The model under review builds one solid part; all positions refer to its coordinate system, in mm. A direction names the side the tool comes from. Coordinates: 2 decimals unless noted, no trailing zeros. Order: outer loops, then holes, each group sorted by start corner. A loop starts at its lowest first (then second) coordinate and runs counter-clockwise, first axis right, second up. Notation, with made-up numbers: M -30.5,2 L -21.5,2 A6 ccw -21.5,9 Z; hole C 81.5,18 d5. An arc over 180 degrees is marked long. One line per item, written item: value.
```python
from build123d import *

# Parameters (mm, degrees)
SKETCH1_W           = 70
SKETCH1_H           = 40
BOSS_EXTRUDE1_DEPTH = 15
SKETCH2_R           = 7.5
CUT_EXTRUDE1_DEPTH  = 56.226805086
SKETCH3_R           = 11.5
CUT_EXTRUDE2_DEPTH  = 16.5
SKETCH4_R           = 2.6
CUT_EXTRUDE3_DEPTH  = 44.011626335
SKETCH5_W           = 10
SKETCH5_H           = 15
BOSS_EXTRUDE2_DEPTH = 3
SKETCH8_W           = 4.25
SKETCH8_H           = 15
BOSS_EXTRUDE5_DEPTH = 10
SKETCH9_W           = 0.6
SKETCH9_H           = 0.6
BOSS_EXTRUDE6_DEPTH = 10


with BuildPart() as part:
    # Sketch1 → Boss-Extrude1 (new body)
    with BuildSketch(Plane.XY):
        Rectangle(SKETCH1_W, SKETCH1_H)
    extrude(amount=BOSS_EXTRUDE1_DEPTH)

    # Sketch2 → Cut-Extrude1 (cut, through all)
    with BuildSketch(Plane.XZ.offset(20)):
        with Locations((-20, 0)):
            Circle(SKETCH2_R)
        with Locations((20, 0)):
            Circle(SKETCH2_R)
    extrude(amount=-CUT_EXTRUDE1_DEPTH, mode=Mode.SUBTRACT)

    # Sketch3 → Cut-Extrude2 (cut, symmetric)
    with BuildSketch(Plane(origin=(0, 0, 0), x_dir=(1, 0, 0), z_dir=(0, 1, 0))):
        with Locations((-20, 0)):
            Circle(SKETCH3_R)
        with Locations((20, 0)):
            Circle(SKETCH3_R)
    extrude(amount=CUT_EXTRUDE2_DEPTH, both=True, mode=Mode.SUBTRACT)

    # Sketch4 → Cut-Extrude3 (cut, through all)
    with BuildSketch(Plane.XY.offset(15)):
        Circle(SKETCH4_R)
    extrude(amount=-CUT_EXTRUDE3_DEPTH, mode=Mode.SUBTRACT)

    # Sketch5 → Boss-Extrude2 (add)
    with BuildSketch(Plane.XY.offset(15)):
        with Locations((-6.1, 12.5)):
            Rectangle(SKETCH5_W, SKETCH5_H)
        with Locations((-6.1, -12.5)):
            Rectangle(SKETCH5_W, SKETCH5_H)
    extrude(amount=BOSS_EXTRUDE2_DEPTH)

    # Sketch8 → Boss-Extrude5 (add)
    with BuildSketch(Plane.XY.offset(18)):
        with Locations((-8.975, 12.5)):
            Rectangle(SKETCH8_W, SKETCH8_H)
        with Locations((-3.225, 12.5)):
            Rectangle(SKETCH8_W, SKETCH8_H)
        with Locations((-8.975, -12.5)):
            Rectangle(SKETCH8_W, SKETCH8_H)
        with Locations((-3.225, -12.5)):
            Rectangle(SKETCH8_W, SKETCH8_H)
    extrude(amount=BOSS_EXTRUDE5_DEPTH)

    # Sketch9 → Boss-Extrude6 (add)
    with BuildSketch(Plane.XY.offset(18)):
        with Locations((-5.65, 19.5)):
            Rectangle(SKETCH9_W, SKETCH9_H)
        with Locations((-5.65, 17.5)):
            Rectangle(SKETCH9_W, SKETCH9_H)
        with Locations((-5.65, 15.5)):
            Rectangle(SKETCH9_W, SKETCH9_H)
        with Locations((-5.65, 13.5)):
            Rectangle(SKETCH9_W, SKETCH9_H)
        with Locations((-5.65, 11.5)):
            Rectangle(SKETCH9_W, SKETCH9_H)
        with Locations((-5.65, 9.5)):
            Rectangle(SKETCH9_W, SKETCH9_H)
        with Locations((-5.65, 7.5)):
            Rectangle(SKETCH9_W, SKETCH9_H)
        with Locations((-5.65, 5.5)):
            Rectangle(SKETCH9_W, SKETCH9_H)
        with Locations((-5.65, -19.5)):
            Rectangle(SKETCH9_W, SKETCH9_H)
        with Locations((-5.65, -17.5)):
            Rectangle(SKETCH9_W, SKETCH9_H)
        with Locations((-5.65, -15.5)):
            Rectangle(SKETCH9_W, SKETCH9_H)
        with Locations((-5.65, -13.5)):
            Rectangle(SKETCH9_W, SKETCH9_H)
        with Locations((-5.65, -11.5)):
            Rectangle(SKETCH9_W, SKETCH9_H)
        with Locations((-5.65, -9.5)):
            Rectangle(SKETCH9_W, SKETCH9_H)
        with Locations((-5.65, -7.5)):
            Rectangle(SKETCH9_W, SKETCH9_H)
        with Locations((-5.65, -5.5)):
            Rectangle(SKETCH9_W, SKETCH9_H)
    extrude(amount=BOSS_EXTRUDE6_DEPTH)


solid = part.part
```
(1) Mouldability with a two-part tool opening along X and no side actions: class faces 1 (the flat face through (20, -16.5, 8)), 2 (the flat face through (-11.1, 12, 21)), 3 (the flat face through (0, -20, 11)) as +X half, -X half, draft (parallel to the pull), parting line (faces both ways), or undercut.
Geometry results:
face 1: undercut
face 2: -X half
face 3: draft
(2) Insertion check: pin 1 Ø5 at (y, z) = (-7, 25) entering from +X; pin 2 Ø0.7 at (x, z) = (-5.5, 25.5) entering from +Y; pin 3 Ø10 at (x, y) = (23, -4) entering from +Z; pin 4 Ø12 at (y, z) = (14, 25) entering from -X. Each pin has a flat end and moves straight along its axis. Give the tip position at first contact, or say it passes through.
Geometry results:
pin 1: stops at x = -1.1
pin 2: stops at y = 20
pin 3: stops at z = 15
pin 4: stops at x = -11.1
(3) We need section C-C, the plane y = -14.5. State the section outline as (x, z) points.
Geometry results:
outline: M -35,0 L -31.5,0 A11.5 cw -8.5,0 L 8.5,0 A11.5 cw 31.5,0 L 35,0 L 35,15 L -1.1,15 L -1.1,28 L -5.35,28 L -5.35,18 L -6.85,18 L -6.85,28 L -11.1,28 L -11.1,15 L -35,15 Z
(4) We need section A-A, the plane y = 1. State the section outline as (x, z) points.
Geometry results:
outline: M -35,0 L -31.5,0 A11.5 cw -8.5,0 L -2.4,0 L -2.4,15 L -35,15 Z; M 2.4,0 L 8.5,0 A11.5 cw 31.5,0 L 35,0 L 35,15 L 2.4,15 Z
(5) We need section B-B, the plane x = 0. State the section outline as (y, z) points, plus the area to 3 significant figures.
Geometry results:
outline: M -20,0 L -2.6,0 L -2.6,15 L -20,15 Z; M 2.6,0 L 20,0 L 20,15 L 2.6,15 Z
area: 522 mm2
(6) We need section D-D, the plane x = 20. State the section outline as (y, z) points.
Geometry results:
outline: M -20,7.5 L -16.5,7.5 L -16.5,11.5 L 16.5,11.5 L 16.5,7.5 L 20,7.5 L 20,15 L -20,15 Z
(7) For L1, parallel to Y at x = 0, z = 8; L2, parallel to Y at x = -17, z = 7; L3, parallel to X at y = 0.5, z = 10.5, list the stretches that pass through material, from the lowest coordinate up.
Geometry results:
L1: y = -20 to -2.6, 2.6 to 20
L2: y = -20 to -16.5, 16.5 to 20
L3: x = -35 to -24.69, -15.31 to -2.55, 2.55 to 15.31, 24.69 to 35
(8) Tool access review of faces 4 (the flat face through (-5.35, -15, 23)), 5 (the flat face through (-5, 5, 21)), 6 (the flat face through (-20, -16.5, 8)): name each direction out of +Z, -Z, +X, -X, +Y, -Y from which nothing blocks a thin tool from reaching the whole face with its end or side.
Geometry results:
face 4: +Z
face 5: +Z, +X, -X
face 6: -Z
